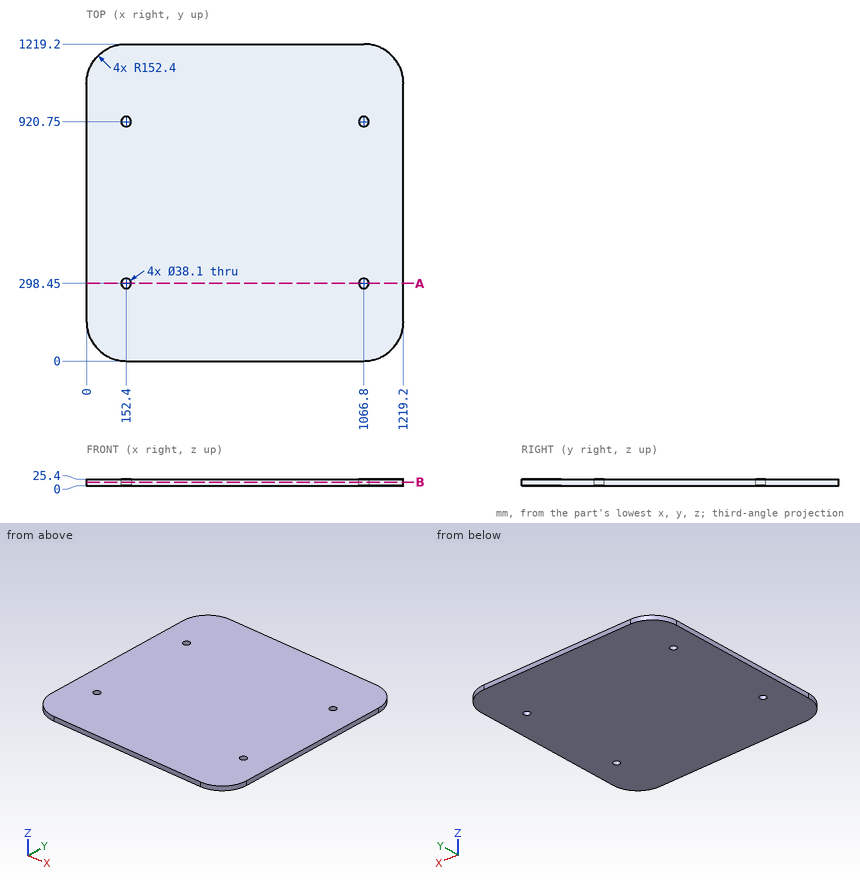
Answer from the drawing. Dimensions are ordinates in mm from the lowest x, y and z of the part. Give positions to 0.01 mm unless a question says otherwise; leave off trailing zeros. Write each loop counter-clockwise with the first axis right and the second up, starting at its lowest first coordinate (ties: lowest second). Pieces come first, ordered by that corner, then holes.
1) Section A-A (y = 298.45) is taken. Write down the section's boundary in (x, z).
2) Section B-B (z = 13) is taken. Write down the section's boundary in (x, y), and give its area (3 significant figures).
3) Find the intervals of material crossed by L1, parallel to Y at x = 152.4, z = 12.5; L2, parallel to Y at x = 79.5, z = 8, in increasing order.
Response:
1. outline: (0, 0) - (133.35, 0) - (133.35, 25.4) - (0, 25.4) - close; (171.45, 0) - (1047.75, 0) - (1047.75, 25.4) - (171.45, 25.4) - close; (1085.85, 0) - (1219.2, 0) - (1219.2, 25.4) - (1085.85, 25.4) - close
2. outline: (0, 152.4) arc R152.4 ccw to (152.4, 0) - (1066.8, 0) arc R152.4 ccw to (1219.2, 152.4) - (1219.2, 1066.8) arc R152.4 ccw to (1066.8, 1219.2) - (152.4, 1219.2) arc R152.4 ccw to (0, 1066.8) - close; hole circle Ø38.1 at (152.4, 298.45); hole circle Ø38.1 at (152.4, 920.75); hole circle Ø38.1 at (1066.8, 298.45); hole circle Ø38.1 at (1066.8, 920.75)
2. area: 1,460,000 mm2
3. L1: y = 0 to 279.4, 317.5 to 901.7, 939.8 to 1219.2
3. L2: y = 18.57 to 1200.63
